The listing builds one solid part. Answer for the finished solid, in the listing's coordinates (mm). A direction names the side the tool comes from. Give positions to 0.01 mm unless a question says otherwise; leave off trailing zeros. Order: outer loops, then holes, each group sorted by start corner. A loop starts at its lowest first (then second) coordinate and runs counter-clockwise, first axis right, second up.
```python
from build123d import *

# Parameters (mm, degrees)
F1_DEPTH = 2.54
F2_R     = 33.02
F3_DEPTH = 1.27
F4_R     = 31.75
F5_DEPTH = 1.016


with BuildPart() as f1:
    # F0 (on Top) → F1 (new body)
    with BuildSketch(Plane.XY):
        Polygon((-4.502899, -44.45), (36.24338, -26.124625), (40.746279, 18.325375), (4.502899, 44.45), (-36.24338, 26.124625), (-40.746279, -18.325375), align=None)
    extrude(amount=F1_DEPTH)

    # F2 (on face) → F3 (cut)
    with BuildSketch(Plane.XY.offset(2.54)):
        Circle(F2_R)
    extrude(amount=-F3_DEPTH, mode=Mode.SUBTRACT)

    # F4 (on face) → F5 (join)
    with BuildSketch(Plane(origin=(0, 0, 0), x_dir=(1, 0, 0), z_dir=(0, 0, -1))):
        Circle(F4_R)
    extrude(amount=F5_DEPTH)


solid = f1.part
```
1) A tool of negligible diameter and unlimited length cuts with its end or side. For faces 1 (the flat face through (6, -33, 2.54)), 2 (the flat face through (0, 0, 1.27)), 3 (the cylindrical face through (-6.883, 30.995, -0.501)), from which of +Z, -Z, +X, -X, +Y, -Y can it reach the whole face along a straight path? Write none if from no direction.
Geometry says:
face 1: +Z, +X, -X, +Y, -Y
face 2: +Z
face 3: -Z
2) Find section A-A (x = -9). Write down the section's boundary in (y, z), then the cut area to 3 significant figures.
Geometry says:
outline: (-41.21, 0) - (-30.45, 0) - (-30.45, -1.02) - (30.45, -1.02) - (30.45, 0) - (38.38, 0) - (38.38, 2.54) - (31.77, 2.54) - (31.77, 1.27) - (-31.77, 1.27) - (-31.77, 2.54) - (-41.21, 2.54) - close
area: 183 mm2
3) For a pull along Y with two mould halves and no side action, classify faces 4 (the flat face through (-15.585, 35.416, 1.252)), 5 (the flat face through (0, 0, -1.016)), 6 (the cylindrical face through (31.5, 9.9, 1.9)) as +Y half, -Y half, draft (parallel to the pull), parting line (faces both ways), or undercut.
Geometry says:
face 4: +Y half
face 5: draft
face 6: undercut
4) Find section B-B (y = 12.5). Write down the section's boundary in (x, z), then the cut area to 3 significant figures.
Geometry says:
outline: (-37.62, 0) - (-29.19, 0) - (-29.19, -1.02) - (29.19, -1.02) - (29.19, 0) - (40.16, 0) - (40.16, 2.54) - (30.56, 2.54) - (30.56, 1.27) - (-30.56, 1.27) - (-30.56, 2.54) - (-37.62, 2.54) - close
area: 179 mm2
5) Straight lines are drawn through the part: probe 1 along Z at (x, y) = (-1, -25.5); probe 2 along Y at (x, z) = (0, 2.2); probe 3 along X at (y, z) = (20, 1.7). For each, find the intervals that lie inside material, in ascending order.
Geometry says:
probe 1: z = -1.02 to 1.27
probe 2: y = -42.42 to -33.02, 33.02 to 42.42
probe 3: x = -36.86 to -26.27, 26.27 to 38.42
6) Find section D-D (y = -36). Write down the section's boundary in (x, z).
Geometry says:
outline: (-16.23, 0) - (14.29, 0) - (14.29, 2.54) - (-16.23, 2.54) - close
7) Given P1, Ø1.5, axis at y = -19.5, z = 2, coming from the +X side; P2, Ø1, axis at x = 17.5, y = 27, coming from the +Z side; P3, Ø2, axis at x = -30, y = -20, coming from the -Z side, each flat-ended and moving along its own axis, determine where each tip first touches the part or whether it passes through.
Geometry says:
P1: stops at x = 36.99
P2: stops at z = 1.27
P3: stops at z = 0
8) Find section C-C (x = 34). Write down the section's boundary in (y, z).
Geometry says:
outline: (-27.13, 0) - (23.19, 0) - (23.19, 2.54) - (-27.13, 2.54) - close
